```python
from build123d import *

# Parameters (mm, degrees)
F0_R     = 22.86
F0_R_2   = 13.49375
F1_DEPTH = 3.175
F2_R     = 2.38125
F3_DEPTH = 25.4


with BuildPart() as f1:
    # F0 (on Top) → F1 (new body)
    with BuildSketch(Plane.XY):
        Circle(F0_R)
        Circle(F0_R_2, mode=Mode.SUBTRACT)
    extrude(amount=F1_DEPTH)

    # F2 (on face) → F3 (cut)
    with BuildSketch(Plane.XY.offset(3.175)):
        with BuildLine():
            ThreePointArc((2.38125, 18.176875), (1.683798, 19.860673), (0, 20.558125))
            Line((0, 20.558125), (0, 15.795625))
            ThreePointArc((0, 15.795625), (1.683798, 16.493077), (2.38125, 18.176875))
        make_face()
        with BuildLine():
            Line((0, 15.795625), (0, 20.558125))
            ThreePointArc((0, 20.558125), (-2.38125, 18.176875), (0, 15.795625))
        make_face()
        with Locations((-18.176875, 0)):
            Circle(F2_R)
        with Locations((0, -18.176875)):
            Circle(F2_R)
        with Locations((18.176875, 0)):
            Circle(F2_R)
    extrude(amount=-F3_DEPTH, mode=Mode.SUBTRACT)


solid = f1.part
```
Input: part model. Units: mm. Frame: model coordinates. Coordinates: 2 decimals unless noted, no trailing zeros. Loops run counter-clockwise (first coordinate to the right, second up) from the corner with the lowest first, then second, coordinate; pieces in that order, holes last.
Q1. Mould query, pull axis X, two halves, no side actions, for faces 1 (the cylindrical face through (-9.945, 9.12, 1.565)), 2 (the flat face through (10, -10, 3.175)), 3 (the cylindrical face through (21.804, 6.867, 1.565)). Classes: +X half, -X half, draft (parallel to the pull), parting line (faces both ways), or undercut.
Results are:
face 1: undercut
face 2: draft
face 3: parting line
Q2. Line query: line 1 along Y through (x, z) = (0, 1.95); line 2 along Y through (x, z) = (-19, 2.2); line 3 along X through (y, z) = (18, 1.2). Output: solid intervals per line, ascending.
Results are:
line 1: y = -22.86 to -20.56, -15.8 to -13.49, 13.49 to 15.8, 20.56 to 22.86
line 2: y = -12.71 to -2.23, 2.23 to 12.71
line 3: x = -14.09 to -2.37, 2.37 to 14.09
Q3. Section B-B, the plane x = -9. Return the cut outline in (y, z) (3 decimals).
Results are:
outline: (-21.014, 0) - (-10.054, 0) - (-10.054, 3.175) - (-21.014, 3.175) - close; (10.054, 0) - (21.014, 0) - (21.014, 3.175) - (10.054, 3.175) - close
Q4. Section D-D, the plane x = 4. Return the cut outline in (y, z) (3 decimals), and give its area (3 significant figures).
Results are:
outline: (-22.507, 0) - (-12.887, 0) - (-12.887, 3.175) - (-22.507, 3.175) - close; (12.887, 0) - (22.507, 0) - (22.507, 3.175) - (12.887, 3.175) - close
area: 61.1 mm2
Q5. Section C-C, the plane z = 1.95. Return the cut outline in (x, y).
Results are:
outline: circle Ø45.72 at (0, 0); hole circle Ø4.76 at (-18.18, 0); hole circle Ø26.99 at (0, 0); hole circle Ø4.76 at (0, -18.18); hole circle Ø4.76 at (0, 18.18); hole circle Ø4.76 at (18.18, 0)
Q6. Section A-A, the plane y = 0. Return the cut outline in (x, z) (3 decimals).
Results are:
outline: (-22.86, 0) - (-20.558, 0) - (-20.558, 3.175) - (-22.86, 3.175) - close; (-15.796, 0) - (-13.494, 0) - (-13.494, 3.175) - (-15.796, 3.175) - close; (13.494, 0) - (15.796, 0) - (15.796, 3.175) - (13.494, 3.175) - close; (20.558, 0) - (22.86, 0) - (22.86, 3.175) - (20.558, 3.175) - close
